The listing builds one solid part. Answer for the finished solid, in the listing's coordinates (mm). A direction names the side the tool comes from. Give positions to 0.01 mm unless a question says otherwise; leave off trailing zeros. Write each loop counter-clockwise with the first axis right and the second up, starting at its lowest first coordinate (ties: lowest second). Pieces come first, ordered by that corner, then holes. Notation, with made-up numbers: (87.5, 47.5) - (94.5, 47.5) arc R32 ccw to (94.5, 82.5) - close; hole circle Ø4 at (61, -29.5). An arc over 180 degrees is marked (long way). Answer as CSV lines item,"result". Start each with the question number.
(1) Straight lines are drawn through the part: probe 1 along Z at (x, y) = (-31, 6.2); probe 2 along Z at (x, y) = (-31, 2.3); probe 3 along X at (y, z) = (6.5, -19). For each, find the intervals that lie inside material, in ascending order.
(2) Find section A-A (x = -31). Write down the section's boundary in (y, z).
(3) Each of these flat-tipped pins is pushed along its axis until it touches: pin 1 Ø1.3 at (x, z) = (15.5, 55) entering from +Y; pin 2 Ø5 at (x, z) = (-23.5, 8) entering from +Y; pin 3 Ø6.5 at (x, z) = (30.5, 54.5) entering from +Y; pin 4 Ø1.7 at (x, z) = (29.5, -54.5) entering from +Y. Where does it stop, or does it pass through?
(4) Find section B-B (x = 19.5). Write down the section's boundary in (y, z).
(5) For faces 1 (the face through (-30, 4, 57)), 2 (the face through (-1, 0, -1)), determine the directions among +Z, -Z, +X, -X, +Y, -Y from which every point of the face is accessible in a straight line to the end or side of a thin tool.
(6) For a pull along Z with two mould halves and no side action, classify faces 3 (the face through (-46.359, 3.549, 57.797)), 4 (the face through (-16, 1, -56)), 5 (the face through (-47.5, 3, 1)) as pulls with the +Z half, pulls with the -Z half, needs draft (parallel to the pull), parting line crosses it, or undercut.
(7) Find section C-C (z = -30). Write down the section's boundary in (x, y).
from build123d import *

# Parameters (mm, degrees)
SZKIC1_W                    = 95
SZKIC1_H                    = 118
DODANIE_WYCI_GNI_CIE1_DEPTH = 7
SZKIC2_W                    = 91.5
SZKIC2_H                    = 104
WYTNIJ_WYCI_GNI_CIE1_DEPTH  = 4
SZKIC4_R                    = 1.6
WYTNIJ_WYCI_GNI_CIE3_DEPTH  = 8
ZAOKR_GLENIE1_R             = 4
SZKIC5_R                    = 2.9
WYTNIJ_WYCI_GNI_CIE4_DEPTH  = 3
SZKIC6_R                    = 2.1
WYTNIJ_WYCI_GNI_CIE5_DEPTH  = 6


with BuildPart() as part:
    # Szkic1 → Dodanie-wyciągnięcie1 (new body)
    with BuildSketch(Plane(origin=(0, 0, 0), x_dir=(1, 0, 0), z_dir=(0, 1, 0))):
        Rectangle(SZKIC1_W, SZKIC1_H)
    extrude(amount=DODANIE_WYCI_GNI_CIE1_DEPTH)

    # Szkic2 → Wytnij-wyciągnięcie1 (cut)
    with BuildSketch(Plane(origin=(0, 7, 0), x_dir=(1, 0, 0), z_dir=(0, 1, 0))):
        Rectangle(SZKIC2_W, SZKIC2_H)
    extrude(amount=-WYTNIJ_WYCI_GNI_CIE1_DEPTH, mode=Mode.SUBTRACT)

    # Szkic4 → Wytnij-wyciągnięcie3 (cut, through all)
    with BuildSketch(Plane(origin=(0, 7, 0), x_dir=(1, 0, 0), z_dir=(0, 1, 0))):
        with Locations((31, -55.5)):
            Circle(SZKIC4_R)
        with Locations((-31, -55.5)):
            Circle(SZKIC4_R)
        with Locations((31, 55.5)):
            Circle(SZKIC4_R)
        with Locations((-31, 55.5)):
            Circle(SZKIC4_R)
    extrude(amount=-WYTNIJ_WYCI_GNI_CIE3_DEPTH, mode=Mode.SUBTRACT)

    # Zaokrąglenie1
    zaokr_glenie1_edges = [part.edges().sort_by_distance(p)[0] for p in [
        (47.5, 3.5, 59),
        (-47.5, 3.5, 59),
        (-47.5, 3.5, -59),
        (47.5, 3.5, -59),
    ]]
    fillet(zaokr_glenie1_edges, radius=ZAOKR_GLENIE1_R)

    # Szkic5 → Wytnij-wyciągnięcie4 (cut)
    with BuildSketch(Plane(origin=(0, 7, 0), x_dir=(1, 0, 0), z_dir=(0, 1, 0))):
        with Locations((-31, -55.5)):
            Circle(SZKIC5_R)
        with Locations((-31, 55.5)):
            Circle(SZKIC5_R)
        with Locations((31, -55.5)):
            Circle(SZKIC5_R)
        with Locations((31, 55.5)):
            Circle(SZKIC5_R)
    extrude(amount=-WYTNIJ_WYCI_GNI_CIE4_DEPTH, mode=Mode.SUBTRACT)

    # Szkic6 → Wytnij-wyciągnięcie5 (cut)
    with BuildSketch(Plane(origin=(0, 7, 0), x_dir=(1, 0, 0), z_dir=(0, 1, 0))):
        with Locations((-16, -55.5)):
            Circle(SZKIC6_R)
        with Locations((-16, 55.5)):
            Circle(SZKIC6_R)
        with Locations((16, 55.5)):
            Circle(SZKIC6_R)
        with Locations((16, -55.5)):
            Circle(SZKIC6_R)
    extrude(amount=-WYTNIJ_WYCI_GNI_CIE5_DEPTH, mode=Mode.SUBTRACT)


solid = part.part
Result set:
1,probe 1,"-59 to -58.4, -52.6 to -52, 52 to 52.6, 58.4 to 59"
1,probe 2,"-59 to -57.1, -53.9 to 53.9, 57.1 to 59"
1,probe 3,"-47.5 to -45.75, 45.75 to 47.5"
2,outline,"(0, -59) - (7, -59) - (7, -58.4) - (4, -58.4) - (4, -57.1) - (0, -57.1) - close; (0, -53.9) - (4, -53.9) - (4, -52.6) - (7, -52.6) - (7, -52) - (3, -52) - (3, 52) - (7, 52) - (7, 52.6) - (4, 52.6) - (4, 53.9) - (0, 53.9) - close; (0, 57.1) - (4, 57.1) - (4, 58.4) - (7, 58.4) - (7, 59) - (0, 59) - close"
3,pin 1,"y = 1"
3,pin 2,"y = 3"
3,pin 3,"y = 7"
3,pin 4,"y = 4"
4,outline,"(0, -59) - (7, -59) - (7, -52) - (3, -52) - (3, 52) - (7, 52) - (7, 59) - (0, 59) - close"
5,face 1,"+Y"
5,face 2,"+Z, -Z, +X, -X, -Y"
6,face 3,"pulls with the +Z half"
6,face 4,"undercut"
6,face 5,"needs draft"
7,outline,"(-47.5, 0) - (47.5, 0) - (47.5, 7) - (45.75, 7) - (45.75, 3) - (-45.75, 3) - (-45.75, 7) - (-47.5, 7) - close"
